from build123d import *

# Parameters (mm, degrees)
F0_W     = 92.71
F0_H     = 57.15
F1_DEPTH = 66.04
F2_T     = -2.54
F4_DEPTH = 25.4
F6_DEPTH = 25.4


with BuildPart() as f1:
    # F0 (on Top) → F1 (new body)
    with BuildSketch(Plane.XY):
        with Locations((46.355, 28.575)):
            Rectangle(F0_W, F0_H)
    extrude(amount=F1_DEPTH)

    # F2
    f2_openings = [f1.faces().sort_by_distance(p)[0] for p in [
        (46.355, 28.575, 66.04),
    ]]
    offset(amount=F2_T, openings=f2_openings)

    # F3 (on face) → F4 (cut)
    with BuildSketch(Plane.XZ):
        with BuildLine():
            Line((56.342959, 66.04), (36.00914, 66.04))
            ThreePointArc((36.00914, 66.04), (46.17605, 50.051373), (56.342959, 66.04))
        make_face()
    extrude(amount=-F4_DEPTH, mode=Mode.SUBTRACT)

    # F5 (on face) → F6 (cut)
    with BuildSketch(Plane.XZ):
        with BuildLine():
            Line((36.00914, 66.04), (25.135325, 66.04))
            ThreePointArc((25.135325, 66.04), (47.225845, 33.909376), (69.316365, 66.04))
            Line((69.316365, 66.04), (56.342959, 66.04))
            ThreePointArc((56.342959, 66.04), (46.17605, 50.051373), (36.00914, 66.04))
        make_face()
    extrude(amount=-F6_DEPTH, mode=Mode.SUBTRACT)


solid = f1.part
Design review of the part built by this model. Coordinates are the model's own, in mm. A direction names the side the tool comes from. Give positions to 0.01 mm unless a question says otherwise; leave off trailing zeros. Loops run counter-clockwise (first coordinate to the right, second up) from the corner with the lowest first, then second, coordinate; pieces in that order, holes last. Notation, with made-up numbers: (10, 4.25) - (39, 4.25) arc R35 ccw to (39, 43.25) - close; hole circle Ø5 at (6, 24.5). An arc over 180 degrees is marked (long way). Write item = value, one per line.
1) Tool access review of faces 4 (the face through (46, 29, 2.54)), 5 (the face through (46, 56, 66.04)): name each direction out of +Z, -Z, +X, -X, +Y, -Y from which nothing blocks a thin tool from reaching the whole face with its end or side.
Result sheet:
face_4 = +Z
face_5 = +Z, +X, -X, +Y, -Y
2) Take a section at C-C on x = 84. State the section outline as (y, z) points, and give its area (3 significant figures).
Result sheet:
outline = (0, 0) - (57.15, 0) - (57.15, 66.04) - (54.61, 66.04) - (54.61, 2.54) - (2.54, 2.54) - (2.54, 66.04) - (0, 66.04) - close
area = 468 mm2
3) To check wall thickness, follow line 1 (X direction, y = 24, z = 50); line 2 (Y direction, x = 33.5, z = 11); line 3 (Y direction, x = 58, z = 58). State the ranges of each line that lie inside material, in increasing order.
Result sheet:
line_1 = 0 to 2.54, 90.17 to 92.71
line_2 = 0 to 2.54, 54.61 to 57.15
line_3 = 54.61 to 57.15
4) Clearance check with a flat-ended pin moving along its axis: pin 1 Ø3 at (x, y) = (32.5, 7) entering from +Z. State where the tip first meets the part, or that it passes through.
Result sheet:
pin_1 = 2.54
5) Take a section at B-B on z = 13. State the section outline as (x, y) points, and give its area (3 significant figures).
Result sheet:
outline = (0, 0) - (92.71, 0) - (92.71, 57.15) - (0, 57.15) - close; hole (2.54, 2.54) - (90.17, 2.54) - (90.17, 54.61) - (2.54, 54.61) - close
area = 735 mm2
6) Take a section at D-D on z = 59. State the section outline as (x, y) points.
Result sheet:
outline = (0, 0) - (23.61, 0) - (23.61, 2.54) - (2.54, 2.54) - (2.54, 54.61) - (90.17, 54.61) - (90.17, 2.54) - (70.84, 2.54) - (70.84, 0) - (92.71, 0) - (92.71, 57.15) - (0, 57.15) - close
7) Draft analysis for pull direction X (two halves, no side actions). For faces 1 (the face through (46, 57.15, 33)), 2 (the face through (92.71, 28, 33)), 3 (the face through (46.58, 1.25, 33.92)), state which applies: +X half, -X half, draft (parallel to the pull), parting line (faces both ways), or undercut.
Result sheet:
face_1 = draft
face_2 = +X half
face_3 = undercut
8) Take a section at A-A on y = 4. State the section outline as (x, z) points, and give its area (3 significant figures).
Result sheet:
outline = (0, 0) - (92.71, 0) - (92.71, 66.04) - (90.17, 66.04) - (90.17, 2.54) - (2.54, 2.54) - (2.54, 66.04) - (0, 66.04) - close
area = 558 mm2
